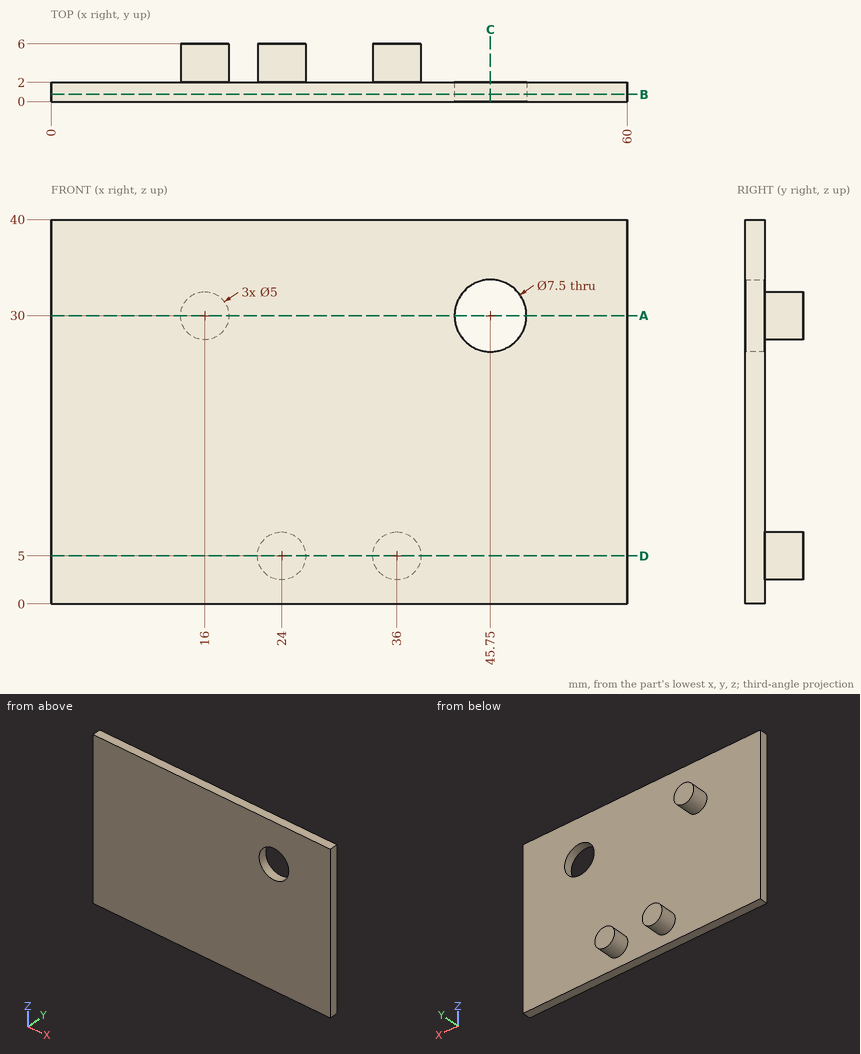
The figure shows three views and two pictorial views of one solid part (mm, origin at its lowest corner). Answer the questions. Coordinates: 2 decimals unless noted, no trailing zeros. Loops run counter-clockwise (first coordinate to the right, second up) from the corner with the lowest first, then second, coordinate; pieces in that order, holes last. Notation, with made-up numbers: (85, 48) -> (102, 48) arc R18 cw to (102, 62) -> close; hole circle Ø9 at (31, -17). An arc over 180 degrees is marked (long way). Write item = value, one per line. Start each with the question number.
1) Straight lines are drawn through the part: line 1 (X direction, y = 0.4, z = 30); line 2 (Z direction, x = 45.75, y = 1.35); line 3 (Y direction, x = 29, z = 32.5). For each, find the intervals that lie inside material, in ascending order. Write a range as from..to.
2) A cutting plane is placed at C-C (x = 45.75). Give the vertices of the cut face in (y, z).
3) A cutting plane is placed at A-A (z = 30). Give the vertices of the cut face in (x, y), then the cut area to 3 significant figures.
4) A cutting plane is placed at D-D (z = 5). Give the vertices of the cut face in (x, y).
5) Given pin 1 Ø12 at (x, z) = (24, 20) entering from +Y, flat-ended and moving along its own axis, determine where the tip first touches the part or whether it passes through.
6) A cutting plane is placed at B-B (y = 0.75). Give the vertices of the cut face in (x, z), then the cut area to 3 significant figures.
Responses:
q1.line_1 = 0..42, 49.5..60
q1.line_2 = 0..26.25, 33.75..40
q1.line_3 = 0..2
q2.outline = (0, 0) -> (2, 0) -> (2, 26.25) -> (0, 26.25) -> close; (0, 33.75) -> (2, 33.75) -> (2, 40) -> (0, 40) -> close
q3.outline = (0, 0) -> (42, 0) -> (42, 2) -> (18.5, 2) -> (18.5, 6) -> (13.5, 6) -> (13.5, 2) -> (0, 2) -> close; (49.5, 0) -> (60, 0) -> (60, 2) -> (49.5, 2) -> close
q3.area = 125 mm²
q4.outline = (0, 0) -> (60, 0) -> (60, 2) -> (38.5, 2) -> (38.5, 6) -> (33.5, 6) -> (33.5, 2) -> (26.5, 2) -> (26.5, 6) -> (21.5, 6) -> (21.5, 2) -> (0, 2) -> close
q5.pin_1 = 2
q6.outline = (0, 0) -> (60, 0) -> (60, 40) -> (0, 40) -> close; hole circle Ø7.5 at (45.75, 30)
q6.area = 2,360 mm²
